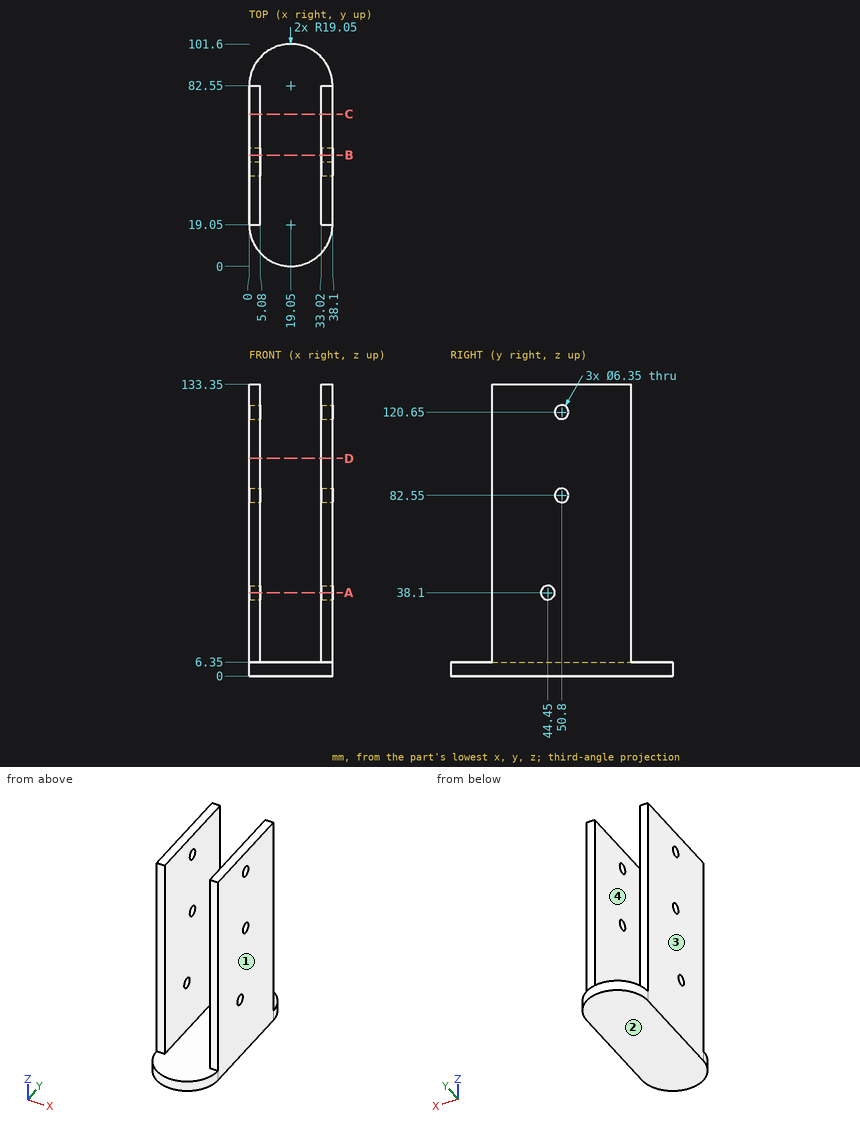
Can you work these out from the drawing? Everything is in mm from the part's minimum corner. Coordinates: 2 decimals unless noted, no trailing zeros. Loops run counter-clockwise (first coordinate to the right, second up) from the corner with the lowest first, then second, coordinate; pieces in that order, holes last. Notation, with made-up numbers: (69, 28.5) - (121, 28.5) arc R23 ccw to (121, 58.5) - close; hole circle Ø8 at (-3, -24). An arc over 180 degrees is marked (long way). Answer as CSV lines item,"result".
Q1. We'd pull the mould along X, two halves only. Please class the marked faces 1, 2, 3 and 4: pulls with the +X half, pulls with the -X half, needs draft (parallel to the pull), parting line crosses it, or undercut.
Response:
face 1,"pulls with the +X half"
face 2,"needs draft"
face 3,"pulls with the -X half"
face 4,"undercut"
Q2. If we section it at C-C, the plane y = 69.5: Write out the boundary of the cut face in (x, z).
Response:
outline,"(0, 0) - (38.1, 0) - (38.1, 133.35) - (33.02, 133.35) - (33.02, 6.35) - (5.08, 6.35) - (5.08, 133.35) - (0, 133.35) - close"
Q3. If we section it at D-D, the plane z = 99.5: Write out the boundary of the cut face in (x, y), and give its area (3 significant figures).
Response:
outline,"(0, 19.05) - (5.08, 19.05) - (5.08, 82.55) - (0, 82.55) - close; (33.02, 19.05) - (38.1, 19.05) - (38.1, 82.55) - (33.02, 82.55) - close"
area,"645 mm2"
Q4. For pin 1 (1.5 mm diameter, centred on x = 35.5, z = 88, fed in from -Y); pin 2 (5 mm diameter, centred on y = 50.8, z = 82.55, fed in from -X); pin 3 (5.5 mm diameter, centred on x = 1.5, z = 49, fed in from +Y); pin 4 (4 mm diameter, centred on x = 25, y = 58, fed in from +Z), each with a flat end and sliding along its axis, tell me the tip position at first contact or that it passes through.
Response:
pin 1,"y = 19.05"
pin 2,"through"
pin 3,"y = 82.55"
pin 4,"z = 6.35"
Q5. If I drill on L1, parallel to X at y = 48, z = 34.5; L2, parallel to Z at x = 36.8, y = 50.8 (3 decimals); L3, parallel to Z at x = 36.05, y = 44.45 (3 decimals), over which ranges is the centre line in solid material (lowest first)? Write a range as [from, to].
Response:
L1,"[0, 5.08], [33.02, 38.1]"
L2,"[0, 79.375], [85.725, 117.475], [123.825, 133.35]"
L3,"[0, 34.925], [41.275, 133.35]"
Q6. If we section it at A-A, the plane z = 38.1: Write out the boundary of the cut face in (x, y) (3 decimals).
Response:
outline,"(0, 19.05) - (5.08, 19.05) - (5.08, 41.275) - (0, 41.275) - close; (0, 47.625) - (5.08, 47.625) - (5.08, 82.55) - (0, 82.55) - close; (33.02, 19.05) - (38.1, 19.05) - (38.1, 41.275) - (33.02, 41.275) - close; (33.02, 47.625) - (38.1, 47.625) - (38.1, 82.55) - (33.02, 82.55) - close"
Q7. If we section it at B-B, the plane y = 50.8: Write out the boundary of the cut face in (x, z) (3 decimals), and give its area (3 significant figures).
Response:
outline,"(0, 0) - (38.1, 0) - (38.1, 79.375) - (33.02, 79.375) - (33.02, 6.35) - (5.08, 6.35) - (5.08, 79.375) - (0, 79.375) - close; (0, 85.725) - (5.08, 85.725) - (5.08, 117.475) - (0, 117.475) - close; (0, 123.825) - (5.08, 123.825) - (5.08, 133.35) - (0, 133.35) - close; (33.02, 85.725) - (38.1, 85.725) - (38.1, 117.475) - (33.02, 117.475) - close; (33.02, 123.825) - (38.1, 123.825) - (38.1, 133.35) - (33.02, 133.35) - close"
area,"1,400 mm2"
